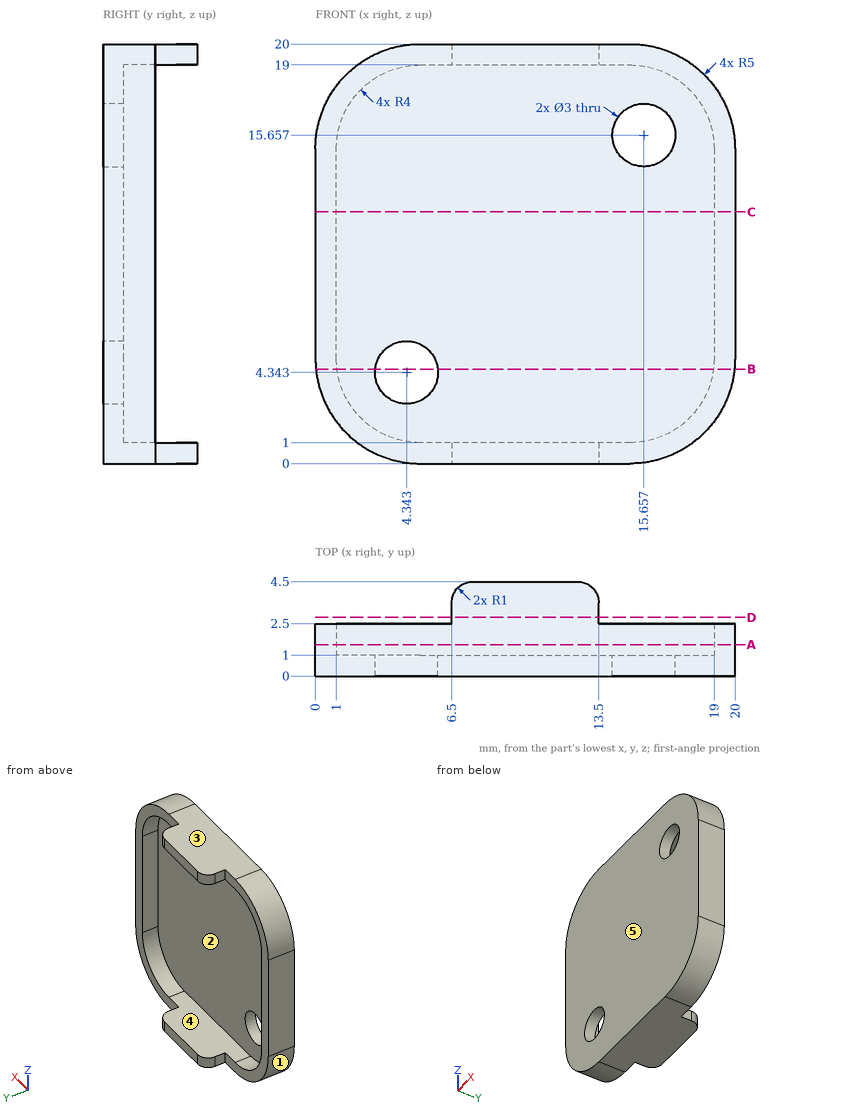
Source: three-view drawing plus pictorial views. Frame: mm from the lowest corner of the part. A direction names the side the tool comes from. Round coordinates to 2 decimals unless told otherwise and drop trailing zeros. Loops run counter-clockwise (first coordinate to the right, second up) from the corner with the lowest first, then second, coordinate; pieces in that order, holes last.
Q1. Access query for the marked faces 4 and 5. Directions: +Z, -Z, +X, -X, +Y, -Y. A direction counts if a zero-diameter tool reaches every point of the face in a straight line with its end or side. Return the directions, or none.
Q2. Ray query, line 1 (Z direction, x = 8.5, y = 4.1); line 2 (Y direction, x = 18.75, z = 15). Return the intervals inside material, ascending.
Q3. Mould query, pull axis X, two halves, no side actions, for the marked faces 1, 2 and 3. Classes: pulls with the +X half, pulls with the -X half, needs draft (parallel to the pull), parting line crosses it, or undercut.
Q4. Section B-B, the plane z = 4.5. Return loops of the section in (x, y) (1 decimal).
Q5. First-contact query: P1, Ø0.8, axis at y = 2, z = 9, coming from the -X side; P2, Ø0.5, axis at y = 3, z = 19.5, coming from the +X side; P3, Ø2.5, axis at x = 4.34, z = 4.34, coming from the -Y side; P4, Ø4, axis at x = 15.66, z = 15.66, coming from the +Y side. Flat tips, straight axial feed; report the tip coordinate or a pass-through.
Q6. Section D-D, the plane y = 2.8. Return loops of the section in (x, z), plus the area to 3 significant figures.
Q7. Section C-C, the plane z = 12. Return loops of the section in (x, y), plus the area to 3 significant figures.
Q8. Section A-A, the plane y = 1.5. Return loops of the section in (x, z).
Solutions:
1. face 4: +Y
1. face 5: +Z, -Z, +X, -X, -Y
2. line 1: z = 0 to 1, 19 to 20
2. line 2: y = 0 to 1
3. face 1: pulls with the -X half
3. face 2: undercut
3. face 3: needs draft
4. outline: (0, 0) - (2.9, 0) - (2.9, 1) - (1, 1) - (1, 2.5) - (0, 2.5) - close; (5.8, 0) - (20, 0) - (20, 2.5) - (19, 2.5) - (19, 1) - (5.8, 1) - close
5. P1: stops at x = 0
5. P2: stops at x = 13.5
5. P3: passes through
5. P4: stops at y = 1
6. outline: (6.5, 0) - (13.5, 0) - (13.5, 1) - (6.5, 1) - close; (6.5, 19) - (13.5, 19) - (13.5, 20) - (6.5, 20) - close
6. area: 14.0 mm2
7. outline: (0, 0) - (20, 0) - (20, 2.5) - (19, 2.5) - (19, 1) - (1, 1) - (1, 2.5) - (0, 2.5) - close
7. area: 23.0 mm2
8. outline: (0, 5) arc R5 ccw to (5, 0) - (15, 0) arc R5 ccw to (20, 5) - (20, 15) arc R5 ccw to (15, 20) - (5, 20) arc R5 ccw to (0, 15) - close; hole (1, 5) arc R4 ccw to (5, 1) - (15, 1) arc R4 ccw to (19, 5) - (19, 15) arc R4 ccw to (15, 19) - (5, 19) arc R4 ccw to (1, 15) - close
